```python
from build123d import *

# Parameters (mm, degrees)
BOSS_EXTRUDE1_DEPTH = 240
CUT_EXTRUDE3_DEPTH  = 245.479549247
BOSS_EXTRUDE2_DEPTH = 240
SKETCH3_R           = 1.625
CUT_EXTRUDE4_DEPTH  = 270
SKETCH3_5_R         = 3.125
SKETCH3_5_R_2       = 1.625
CUT_EXTRUDE5_DEPTH  = 2
CUT_EXTRUDE6_DEPTH  = 245.810237745


with BuildPart() as part:
    # Sketch2 → Boss-Extrude1 (new body)
    with BuildSketch(Plane(origin=(0, 15, 0), x_dir=(1, 0, 0), z_dir=(0, 1, 0))):
        with BuildLine():
            Line((-10, -44.38749824), (-10, -41.306779105))
            ThreePointArc((-10, -41.306779105), (0, -42.5), (10, -41.306779105))
            Line((10, -41.306779105), (10, -44.38749824))
            ThreePointArc((10, -44.38749824), (0, -45.5), (-10, -44.38749824))
        make_face()
    extrude(amount=BOSS_EXTRUDE1_DEPTH)

    # Sketch5 → Cut-Extrude3 (cut, through all)
    with BuildSketch(Plane(origin=(0, 255, 0), x_dir=(1, 0, 0), z_dir=(0, 1, 0))):
        with BuildLine():
            Line((-8, -42.991182168), (-8, -44.791182168))
            ThreePointArc((-8, -44.791182168), (-9.002263059, -44.600552237), (-10, -44.38749824))
            Line((-10, -44.38749824), (-10, -42.570432746))
            ThreePointArc((-10, -42.570432746), (-9.002458415, -42.792493345), (-8, -42.991182168))
        make_face()
        with BuildLine():
            Line((8, -44.791182168), (8, -42.991182168))
            ThreePointArc((8, -42.991182168), (9.002458415, -42.792493345), (10, -42.570432746))
            Line((10, -42.570432746), (10, -44.38749824))
            ThreePointArc((10, -44.38749824), (9.002263059, -44.600552237), (8, -44.791182168))
        make_face()
    extrude(amount=-CUT_EXTRUDE3_DEPTH, mode=Mode.SUBTRACT)

    # Sketch6 → Boss-Extrude2 (add, through all)
    with BuildSketch(Plane(origin=(0, 255, 0), x_dir=(1, 0, 0), z_dir=(0, 1, 0))):
        with BuildLine():
            Line((-8, -44.791182168), (-8, -46.821469434))
            ThreePointArc((-8, -46.821469434), (-6.468173714, -47.057546991), (-4.929460777, -47.243522481))
            ThreePointArc((-4.929460777, -47.243522481), (-4.736798282, -47.146817981), (-4.743851161, -46.931362988))
            Line((-4.743851161, -46.931362988), (-6, -45.102660675))
            ThreePointArc((-6, -45.102660675), (-7.001732265, -44.958044278), (-8, -44.791182168))
        make_face()
        with BuildLine():
            Line((8, -44.791182168), (8, -46.821469434))
            ThreePointArc((8, -46.821469434), (6.468173714, -47.057546991), (4.929460777, -47.243522481))
            ThreePointArc((4.929460777, -47.243522481), (4.736798282, -47.146817981), (4.743851161, -46.931362988))
            Line((4.743851161, -46.931362988), (6, -45.102660675))
            ThreePointArc((6, -45.102660675), (7.001732265, -44.958044278), (8, -44.791182168))
        make_face()
    extrude(amount=-BOSS_EXTRUDE2_DEPTH)

    # Sketch3 → Cut-Extrude4 (cut)
    with BuildSketch(Plane.XY.offset(45.5)):
        with Locations((0, 30)):
            Circle(SKETCH3_R)
        with Locations((0, 60)):
            Circle(SKETCH3_R)
        with Locations((0, 90)):
            Circle(SKETCH3_R)
        with Locations((0, 120)):
            Circle(SKETCH3_R)
        with Locations((0, 150)):
            Circle(SKETCH3_R)
        with Locations((0, 180)):
            Circle(SKETCH3_R)
        with Locations((0, 210)):
            Circle(SKETCH3_R)
        with Locations((0, 240)):
            Circle(SKETCH3_R)
    extrude(amount=-CUT_EXTRUDE4_DEPTH, mode=Mode.SUBTRACT)

    # Sketch3<5> → Cut-Extrude5 (cut)
    # profile 1 of 8: a face of its own
    with BuildSketch(Plane.XY.offset(45.5)):
        with Locations((0, 30)):
            Circle(SKETCH3_5_R)
        with Locations((0, 30)):
            Circle(SKETCH3_5_R_2, mode=Mode.SUBTRACT)
    # profile 2 of 8: a face of its own
    with BuildSketch(Plane.XY.offset(45.5)):
        with Locations((0, 60)):
            Circle(SKETCH3_5_R)
        with Locations((0, 60)):
            Circle(SKETCH3_5_R_2, mode=Mode.SUBTRACT)
    # profile 3 of 8: a face of its own
    with BuildSketch(Plane.XY.offset(45.5)):
        with Locations((0, 90)):
            Circle(SKETCH3_5_R)
        with Locations((0, 90)):
            Circle(SKETCH3_5_R_2, mode=Mode.SUBTRACT)
    # profile 4 of 8: a face of its own
    with BuildSketch(Plane.XY.offset(45.5)):
        with Locations((0, 120)):
            Circle(SKETCH3_5_R)
        with Locations((0, 120)):
            Circle(SKETCH3_5_R_2, mode=Mode.SUBTRACT)
    # profile 5 of 8: a face of its own
    with BuildSketch(Plane.XY.offset(45.5)):
        with Locations((0, 150)):
            Circle(SKETCH3_5_R)
        with Locations((0, 150)):
            Circle(SKETCH3_5_R_2, mode=Mode.SUBTRACT)
    # profile 6 of 8: a face of its own
    with BuildSketch(Plane.XY.offset(45.5)):
        with Locations((0, 180)):
            Circle(SKETCH3_5_R)
        with Locations((0, 180)):
            Circle(SKETCH3_5_R_2, mode=Mode.SUBTRACT)
    # profile 7 of 8: a face of its own
    with BuildSketch(Plane.XY.offset(45.5)):
        with Locations((0, 210)):
            Circle(SKETCH3_5_R)
        with Locations((0, 210)):
            Circle(SKETCH3_5_R_2, mode=Mode.SUBTRACT)
    # profile 8 of 8: a face of its own
    with BuildSketch(Plane.XY.offset(45.5)):
        with Locations((0, 240)):
            Circle(SKETCH3_5_R)
        with Locations((0, 240)):
            Circle(SKETCH3_5_R_2, mode=Mode.SUBTRACT)
    extrude(amount=-CUT_EXTRUDE5_DEPTH, mode=Mode.SUBTRACT)

    # Sketch8 → Cut-Extrude6 (cut, through all)
    with BuildSketch(Plane(origin=(0, 255, 0), x_dir=(1, 0, 0), z_dir=(0, 1, 0))):
        with BuildLine():
            Line((-7.3, -48.974342188), (-7.3, -43.115562668))
            ThreePointArc((-7.3, -43.115562668), (-8.65429325, -42.86426195), (-10, -42.570432746))
            Line((-10, -42.570432746), (-7.3, -48.974342188))
        make_face()
        with BuildLine():
            Line((7.3, -43.115562668), (7.3, -48.974342188))
            Line((7.3, -48.974342188), (10, -42.570432746))
            ThreePointArc((10, -42.570432746), (8.65429325, -42.86426195), (7.3, -43.115562668))
        make_face()
    extrude(amount=-CUT_EXTRUDE6_DEPTH, mode=Mode.SUBTRACT)


solid = part.part
```
Read the model definition and answer for the solid it produces. Units are mm, in the model's axes. A direction names the side the tool comes from. Give positions to 0.01 mm unless a question says otherwise; leave off trailing zeros. Loops run counter-clockwise (first coordinate to the right, second up) from the corner with the lowest first, then second, coordinate; pieces in that order, holes last.
Item 1: Find the intervals of material crossed by line 1 along X through (y, z) = (180, 44.7) (3 decimals); line 2 along X through (y, z) = (60, 43.2) (3 decimals); line 3 along X through (y, z) = (34, 43.15), in increasing order.
Item 2: The part is cut by section A-A (y = 67.5). Write down the section's boundary in (x, z), and give its area (3 significant figures).
Item 3: For faces 1 (the cylindrical face through (-0.1, 133.3, 42.5)), 2 (the flat face through (-7.3, 137, 45)), 3 (the flat face through (7.3, 137, 45)), 4 (the flat face through (1.3, 28.7, 43.5)), determine the directions among +Z, -Z, +X, -X, +Y, -Y from which every point of the face is accessible in a straight line to the end or side of a thin tool.
Item 4: The mould has two halves that part along Y. Classify faces 5 (the flat face through (0, 255, 44)), 6 (the flat face through (1.3, 178.7, 43.5)), 7 (the cylindrical face through (1.442, 117.228, 44.514)), 8 (the flat face through (0, 15, 44)): released by +Y, released by -Y, zero draft, split by the parting line, or undercut.
Item 5: Each of these flat-tipped pins is pushed along its axis until it touches: pin 1 Ø5 at (x, y) = (0, 150) entering from +Z; pin 2 Ø5 at (x, y) = (-1.5, 240.5) entering from +Z; pin 3 Ø7 at (x, y) = (-1.5, 211) entering from +Z; pin 4 Ø10 at (x, y) = (0, 90) entering from -Z. Where does it stop, or does it pass through?
Taken from the geometry:
1. line 1: x = -7.3 to -3.125, 3.125 to 7.3
1. line 2: x = -7.3 to -1.625, 1.625 to 7.3
1. line 3: x = -7.3 to 7.3
2. outline: (-10, 41.31) arc R42.5 cw to (10, 41.31) - (10, 42.57) arc R43.73 ccw to (7.3, 43.12) - (7.3, 46.94) arc R47.5 ccw to (4.93, 47.24) arc R0.2 ccw to (4.74, 46.93) - (6, 45.1) arc R45.5 ccw to (-6, 45.1) - (-4.74, 46.93) arc R0.2 ccw to (-4.93, 47.24) arc R47.5 ccw to (-7.3, 46.94) - (-7.3, 43.12) arc R43.73 ccw to (-10, 42.57) - close
2. area: 59.0 mm2
3. face 1: -Z, +Y, -Y
3. face 2: +Z, -X, +Y, -Y
3. face 3: +Z, +X, +Y, -Y
3. face 4: +Z
4. face 5: released by +Y
4. face 6: undercut
4. face 7: undercut
4. face 8: released by -Y
5. pin 1: stops at z = 43.5
5. pin 2: stops at z = 45.49
5. pin 3: stops at z = 47.24
5. pin 4: stops at z = 42.2
